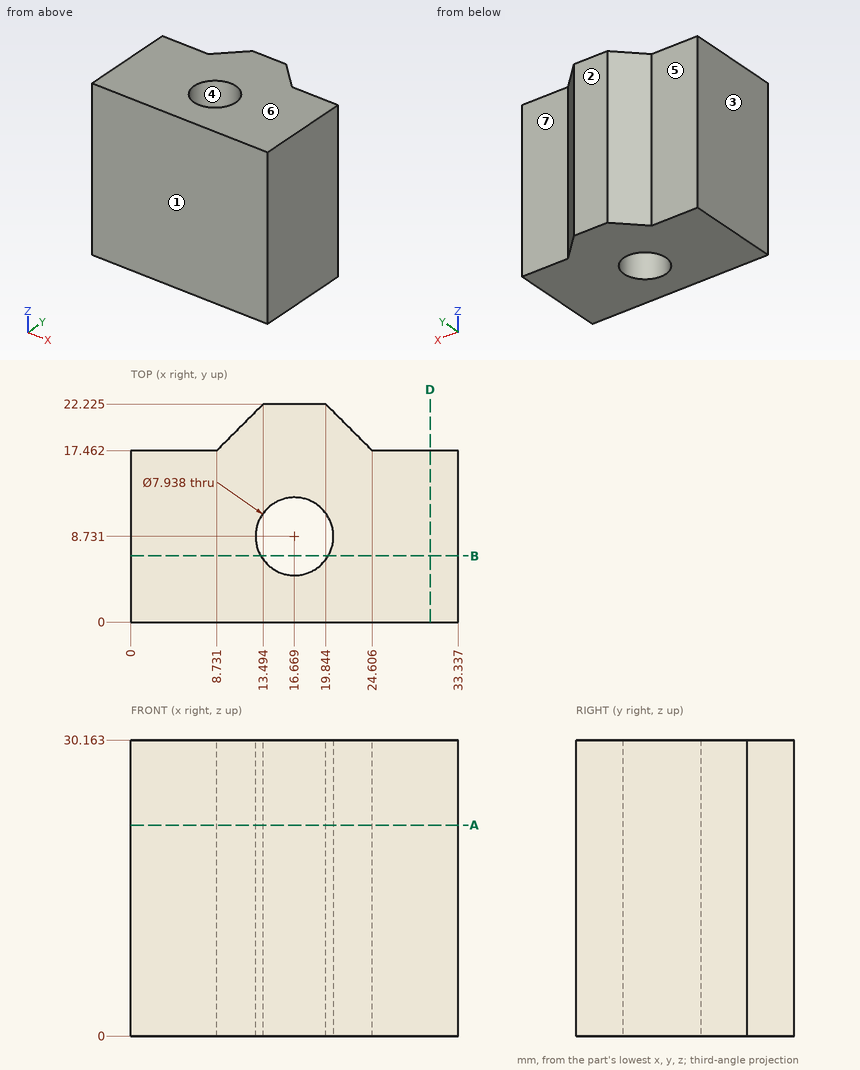
Could you check a few things on this drawing? It's one solid part, dimensions in mm from its lowest x, y, z. A direction names the side the tool comes from. Round coordinates to 2 decimals unless told otherwise and drop trailing zeros. Write each loop counter-clockwise with the first axis right and the second up, starting at its lowest first coordinate (ties: lowest second). Pieces come first, ordered by that corner, then holes. Notation, with made-up numbers: (53, 68) -> (58, 68) arc R13 ccw to (58, 76) -> close; hole circle Ø3 at (39.25, -20). An arc over 180 degrees is marked (long way). Use a Markdown table: item, result.
1. We'd pull the mould along Y, two halves only. Please class the marked faces 1, 2, 3 and 4: +Y half, -Y half, draft (parallel to the pull), parting line (faces both ways), or undercut.
Answer key:
| item | result |
|---|---|
| face 1 | -Y half |
| face 2 | +Y half |
| face 3 | draft |
| face 4 | undercut |
2. Please list where these lines run through material, in increasing order: probe 1 along Y at (x, z) = (27, 9.5); probe 2 along X at (y, z) = (6.75, 28.5); probe 3 along Y at (x, z) = (17, 27) (1 decimal).
Answer key:
| item | result |
|---|---|
| probe 1 | y = 0 to 17.46 |
| probe 2 | x = 0 to 13.23, 20.11 to 33.34 |
| probe 3 | y = 0 to 4.8, 12.7 to 22.2 |
3. Which directions (+Z, -Z, +X, -X, +Y, -Y) give clear straight access to the entire face, cutting with the end or side of a thin tool? Please do the marked faces 5, 6 and 7.
Answer key:
| item | result |
|---|---|
| face 5 | +Z, -Z, -X, +Y |
| face 6 | +Z, +X, -X, +Y, -Y |
| face 7 | +Z, -Z, +X, +Y |
4. For pin 1 Ø7 at (x, z) = (30, 19) entering from +Y; pin 2 Ø2 at (y, z) = (19, 9.5) entering from -X; pin 3 Ø9.5 at (x, z) = (6, 16) entering from +Y, each with a flat end and sliding along its axis, tell me the tip position at first contact or that it passes through.
Answer key:
| item | result |
|---|---|
| pin 1 | stops at y = 17.46 |
| pin 2 | stops at x = 9.27 |
| pin 3 | stops at y = 19.48 |
5. If we section it at D-D (x = 30.5): List the corners of the cut face in (y, z) for me.
Answer key:
| item | result |
|---|---|
| outline | (0, 0) -> (17.46, 0) -> (17.46, 30.16) -> (0, 30.16) -> close |
6. If we section it at B-B (y = 6.75): List the corners of the cut face in (x, z) for me.
Answer key:
| item | result |
|---|---|
| outline | (0, 0) -> (13.23, 0) -> (13.23, 30.16) -> (0, 30.16) -> close; (20.11, 0) -> (33.34, 0) -> (33.34, 30.16) -> (20.11, 30.16) -> close |
7. If we section it at A-A (z = 21.5): List the corners of the cut face in (x, y) for me (1 decimal).
Answer key:
| item | result |
|---|---|
| outline | (0, 0) -> (33.3, 0) -> (33.3, 17.5) -> (24.6, 17.5) -> (19.8, 22.2) -> (13.5, 22.2) -> (8.7, 17.5) -> (0, 17.5) -> close; hole circle Ø7.9 at (16.7, 8.7) |
